CAD build for the part. Positions are in the model's coordinates, mm. Round coordinates to 2 decimals unless told otherwise and drop trailing zeros. Order: outer loops, then holes, each group sorted by start corner. A loop starts at its lowest first (then second) coordinate and runs counter-clockwise, first axis right, second up.
```python
from build123d import *

# Parameters (mm, degrees)
SKETCH2_R           = 1.65
SKETCH2_R_2         = 11
SKETCH2_R_3         = 2.25
SKETCH2_W           = 5
SKETCH2_H           = 5
BOSS_EXTRUDE1_DEPTH = 3.8


with BuildPart() as part:
    # Sketch2 → Boss-Extrude1 (new body)
    with BuildSketch(Plane.XY):
        with BuildLine():
            Line((-155, 155), (-122, 155))
            ThreePointArc((-122, 155), (-120.585786438, 154.414213562), (-120, 153))
            Line((-120, 153), (-120, 145.072545974))
            Line((-120, 145.072545974), (120, 145.072545974))
            Line((120, 145.072545974), (120, 153))
            ThreePointArc((120, 153), (120.585786438, 154.414213562), (122, 155))
            Line((122, 155), (155, 155))
            Line((155, 155), (155, 147.5))
            Line((155, 147.5), (150, 147.5))
            Line((150, 147.5), (150, 142.5))
            Line((150, 142.5), (155, 142.5))
            Line((155, 142.5), (155, 55))
            Line((155, 55), (140, 55))
            Line((140, 55), (140, -5))
            Line((140, -5), (155, -5))
            Line((155, -5), (155, -92.5))
            Line((155, -92.5), (150, -92.5))
            Line((150, -92.5), (150, -97.5))
            Line((150, -97.5), (155, -97.5))
            Line((155, -97.5), (155, -105))
            Line((155, -105), (122, -105))
            ThreePointArc((122, -105), (120.585786438, -104.414213562), (120, -103))
            Line((120, -103), (120, -22))
            ThreePointArc((120, -22), (119.414213562, -20.585786438), (118, -20))
            Line((118, -20), (-118, -20))
            ThreePointArc((-118, -20), (-119.414213562, -20.585786438), (-120, -22))
            Line((-120, -22), (-120, -103))
            ThreePointArc((-120, -103), (-120.585786438, -104.414213562), (-122, -105))
            Line((-122, -105), (-155, -105))
            Line((-155, -105), (-155, -97.5))
            Line((-155, -97.5), (-150, -97.5))
            Line((-150, -97.5), (-150, -92.5))
            Line((-150, -92.5), (-155, -92.5))
            Line((-155, -92.5), (-155, -5))
            Line((-155, -5), (-140, -5))
            Line((-140, -5), (-140, 55))
            Line((-140, 55), (-155, 55))
            Line((-155, 55), (-155, 142.5))
            Line((-155, 142.5), (-150, 142.5))
            Line((-150, 142.5), (-150, 147.5))
            Line((-150, 147.5), (-155, 147.5))
            Line((-155, 147.5), (-155, 155))
        make_face()
        with Locations(Location((-140.309773495, 121.076789794, 0), (0, 0, 180))):
            Circle(SKETCH2_R, mode=Mode.SUBTRACT)
        with Locations(Location((-140.309773495, 92.407184142, 0), (0, 0, 180))):
            Circle(SKETCH2_R, mode=Mode.SUBTRACT)
        with Locations(Location((140.309773495, 121.076789794, 0), (0, 0, 180))):
            Circle(SKETCH2_R, mode=Mode.SUBTRACT)
        with Locations(Location((140.309773495, 92.407184142, 0), (0, 0, 180))):
            Circle(SKETCH2_R, mode=Mode.SUBTRACT)
        with Locations(Location((140.309773495, 106.741986968, 0), (0, 0, 180))):
            Circle(SKETCH2_R_2, mode=Mode.SUBTRACT)
        with Locations(Location((-140.309773495, 106.741986968, 0), (0, 0, 180))):
            Circle(SKETCH2_R_2, mode=Mode.SUBTRACT)
        with Locations(Location((125.59774802, -0.5, 0), (0, 0, 180))):
            Circle(SKETCH2_R, mode=Mode.SUBTRACT)
        with Locations(Location((125.59774802, 50.5, 0), (0, 0, 180))):
            Circle(SKETCH2_R, mode=Mode.SUBTRACT)
        with Locations(Location((-125.59774802, -0.5, 0), (0, 0, 180))):
            Circle(SKETCH2_R, mode=Mode.SUBTRACT)
        with Locations(Location((-125.59774802, 50.5, 0), (0, 0, 180))):
            Circle(SKETCH2_R, mode=Mode.SUBTRACT)
        with Locations(Location((-29, 10.055, 0), (0, 0, 180))):
            Circle(SKETCH2_R_3, mode=Mode.SUBTRACT)
        with Locations(Location((-29, 39.945, 0), (0, 0, 180))):
            Circle(SKETCH2_R_3, mode=Mode.SUBTRACT)
        with Locations(Location((-53.06, 39.945, 0), (0, 0, 180))):
            Circle(SKETCH2_R_3, mode=Mode.SUBTRACT)
        with Locations(Location((-53.06, 10.055, 0), (0, 0, 180))):
            Circle(SKETCH2_R_3, mode=Mode.SUBTRACT)
        with Locations(Location((53.06, 10.055, 0), (0, 0, 180))):
            Circle(SKETCH2_R_3, mode=Mode.SUBTRACT)
        with Locations(Location((29, 10.055, 0), (0, 0, 180))):
            Circle(SKETCH2_R_3, mode=Mode.SUBTRACT)
        with Locations(Location((29, 39.945, 0), (0, 0, 180))):
            Circle(SKETCH2_R_3, mode=Mode.SUBTRACT)
        with Locations(Location((53.06, 39.945, 0), (0, 0, 180))):
            Circle(SKETCH2_R_3, mode=Mode.SUBTRACT)
        with Locations(Location((140.309773495, -71.076789794, 0), (0, 0, 180))):
            Circle(SKETCH2_R, mode=Mode.SUBTRACT)
        with Locations(Location((140.309773495, -42.407184142, 0), (0, 0, 180))):
            Circle(SKETCH2_R, mode=Mode.SUBTRACT)
        with Locations(Location((140.309773495, -56.741986968, 0), (0, 0, 180))):
            Circle(SKETCH2_R_2, mode=Mode.SUBTRACT)
        with Locations(Location((-140.309773495, -56.741986968, 0), (0, 0, 180))):
            Circle(SKETCH2_R_2, mode=Mode.SUBTRACT)
        with Locations(Location((-140.309773495, -42.407184142, 0), (0, 0, 180))):
            Circle(SKETCH2_R, mode=Mode.SUBTRACT)
        with Locations(Location((-140.309773495, -71.076789794, 0), (0, 0, 180))):
            Circle(SKETCH2_R, mode=Mode.SUBTRACT)
        with Locations(Location((38.179918963, -11.563765186, 0), (0, 0, 180))):
            Circle(SKETCH2_R_3, mode=Mode.SUBTRACT)
        with Locations(Location((-38.179918963, -11.563765186, 0), (0, 0, 180))):
            Circle(SKETCH2_R_3, mode=Mode.SUBTRACT)
        with BuildLine():
            Line((-66, 62.171403079), (-111.59774802, 62.171403079))
            ThreePointArc((-111.59774802, 62.171403079), (-114.426175145, 60.999830204), (-115.59774802, 58.171403079))
            Line((-115.59774802, 58.171403079), (-115.59774802, -8.171403079))
            ThreePointArc((-115.59774802, -8.171403079), (-114.426175145, -10.999830204), (-111.59774802, -12.171403079))
            Line((-111.59774802, -12.171403079), (-66, -12.171403079))
            ThreePointArc((-66, -12.171403079), (-63.171572875, -10.999830204), (-62, -8.171403079))
            Line((-62, -8.171403079), (-62, 58.171403079))
            ThreePointArc((-62, 58.171403079), (-63.171572875, 60.999830204), (-66, 62.171403079))
        make_face(mode=Mode.SUBTRACT)
        with BuildLine():
            Line((66, 62.171403079), (111.59774802, 62.171403079))
            ThreePointArc((111.59774802, 62.171403079), (114.426175145, 60.999830204), (115.59774802, 58.171403079))
            Line((115.59774802, 58.171403079), (115.59774802, -8.171403079))
            ThreePointArc((115.59774802, -8.171403079), (114.426175145, -10.999830204), (111.59774802, -12.171403079))
            Line((111.59774802, -12.171403079), (66, -12.171403079))
            ThreePointArc((66, -12.171403079), (63.171572875, -10.999830204), (62, -8.171403079))
            Line((62, -8.171403079), (62, 58.171403079))
            ThreePointArc((62, 58.171403079), (63.171572875, 60.999830204), (66, 62.171403079))
        make_face(mode=Mode.SUBTRACT)
        with Locations((-145, -87.5)):
            Rectangle(SKETCH2_W, SKETCH2_H, mode=Mode.SUBTRACT)
        with Locations((-137.5, -95)):
            Rectangle(SKETCH2_W, SKETCH2_H, mode=Mode.SUBTRACT)
        with Locations((137.5, -95)):
            Rectangle(SKETCH2_W, SKETCH2_H, mode=Mode.SUBTRACT)
        with Locations((145, -87.5)):
            Rectangle(SKETCH2_W, SKETCH2_H, mode=Mode.SUBTRACT)
        with Locations((-137.5, 145)):
            Rectangle(SKETCH2_W, SKETCH2_H, mode=Mode.SUBTRACT)
        with Locations((-145, 137.5)):
            Rectangle(SKETCH2_W, SKETCH2_H, mode=Mode.SUBTRACT)
        with Locations((145, 137.5)):
            Rectangle(SKETCH2_W, SKETCH2_H, mode=Mode.SUBTRACT)
        with Locations((137.5, 145)):
            Rectangle(SKETCH2_W, SKETCH2_H, mode=Mode.SUBTRACT)
    extrude(amount=BOSS_EXTRUDE1_DEPTH)


solid = part.part
```
1. Pin check, flat tips, straight feed: P1, Ø1.9, axis at y = 144, z = 2, coming from the +X side; P2, Ø1.1, axis at x = 100, z = 1, coming from the +Y side. Stop position of each tip, or through.
2. Cut at C-C, the plane y = -34. Write the cut outline in (x, z), and give its area (3 significant figures).
3. Drill centre lines: line 1 (X direction, y = 144, z = 2.55); line 2 (Y direction, x = 29, z = 2.4) (3 decimals); line 3 (X direction, y = 0, z = 0.55). Where is each one in solid material? Low to high.
4. Mould opens along Y. For faces 1 (the face through (-146.223, 97.467, 1.873)), 2 (the face through (2, 56, 3.8)) say: released by +Y, released by -Y, zero draft, split by the parting line, or undercut.
5. Cut at D-D, the plane z = 1.75. Give the number of separate pieces and of enclosed holes in the cut face, and give its area (3 significant figures).
6. Cut at A-A, the plane x = -83. Write the cut outline in (y, z), and give its area (3 significant figures).
7. Cut at B-B, the plane y = 29. Write the cut outline in (x, z), and give its area (3 significant figures).
Outcome:
1. P1: stops at x = 150
1. P2: stops at y = 145.07
2. outline: (-155, 0) - (-120, 0) - (-120, 3.8) - (-155, 3.8) - close; (120, 0) - (155, 0) - (155, 3.8) - (120, 3.8) - close
2. area: 266 mm2
3. line 1: x = -150 to -140, -135 to 135, 140 to 150
3. line 2: y = -20 to 7.805, 12.305 to 37.695, 42.195 to 145.073
3. line 3: x = -140 to -127.17, -124.03 to -115.6, -62 to 62, 115.6 to 124.03, 127.17 to 140
4. face 1: undercut
4. face 2: zero draft
5. separate pieces: 1
5. enclosed holes: 36
5. area: 46,000 mm2
6. outline: (-20, 0) - (-12.17, 0) - (-12.17, 3.8) - (-20, 3.8) - close; (62.17, 0) - (145.07, 0) - (145.07, 3.8) - (62.17, 3.8) - close
6. area: 345 mm2
7. outline: (-140, 0) - (-115.6, 0) - (-115.6, 3.8) - (-140, 3.8) - close; (-62, 0) - (62, 0) - (62, 3.8) - (-62, 3.8) - close; (115.6, 0) - (140, 0) - (140, 3.8) - (115.6, 3.8) - close
7. area: 657 mm2
